Autodesk Inventor part; units mm, degrees
ref_plane "YZ Plane" through (0, 0, 0) normal (1, 0, 0) x (0, 1, 0)
ref_plane "XZ Plane" through (0, 0, 0) normal (0, 1, 0) x (-1, 0, 0)
ref_plane "XY Plane" through (0, 0, 0) normal (0, 0, 1) x (1, 0, 0)
sketch "Sketch1" plane through (0, 0, 0) normal (0, 0, 1) x (1, 0, 0)
  line L0 (1.5658, -2.5487) -> (1.5658, 2.559)
  arc A0 (1.5658, 2.559) -> (1.5824, -2.5487) centre (0, 0) ccw
  line L1 (1.5824, -2.5487) -> (1.5658, -2.5487)
  circle A1 centre (0, 0) radius 10
  circle A2 centre (0, 0) radius 3.1
  line L2 (1.7658, 2.5479) -> (1.7658, -2.5479)
  point P0 (0, 0)
  dimension "d0" = 20
  dimension "d1" = 6.2
  dimension "d2" = 0.2
extrude "Extrusion1" add sketch "Sketch1" against normal blind 10 contours A1 | A2 L2 picked at (2.2105, 0)
sketch "Sketch2" plane through (0, 0, 0) normal (0, 0, 1) x (1, 0, 0)
  circle A0 centre (0, 0) radius 3.1474
  circle A1 centre (0, 0) radius 10
extrude "Extrusion2" add sketch "Sketch2" along normal blind 15
sketch "Sketch3" plane through (0, 0, 15) normal (0, 0, 1) x (1, 0, 0)
  line L0 (7, 1.25) -> (-7, 1.25)
  line L1 (-7, 1.25) -> (-7, -1.25)
  line L2 (-7, -1.25) -> (7, -1.25)
  line L3 (7, -1.25) -> (7, 1.25)
  circle A0 centre (0, 0) radius 10
  dimension "d7" = 2.5
  dimension "d8" = 14
  dimension "d9" = 1.25
  dimension "d10" = 7
extrude "Extrusion3" add sketch "Sketch3" along normal blind 15
properties part number "RollerMotorCoupler"
Build history of the part. All positions in model axes, mm. A direction names the side the tool comes from. Round coordinates to 2 decimals unless told otherwise and drop trailing zeros. Write each loop counter-clockwise with the first axis right and the second up, starting at its lowest first coordinate (ties: lowest second). Pieces come first, ordered by that corner, then holes.
1) Band-saw the part on B-B, the plane x = 0. List the corners of the cut face in (y, z), and give its area (3 significant figures).
2) 3-axis set-ups, long thin cutter, end or side, ignore diameter. For faces 5 (the cylindrical face through (-3.144, -0.138, 7.395)), 6 (the flat face through (0, -1.25, 22)), 7 (the cylindrical face through (-3.1, 0.1, -4.9)): which of +Z, -Z, +X, -X, +Y, -Y reach the whole face in a straight line?
3) Band-saw the part on C-C, the plane z = 19. List the corners of the cut face in (x, y).
4) Band-saw the part on D-D, the plane x = -5. List the corners of the cut face in (y, z).
5) Pin check, flat tips, straight feed: pin 1 (12 mm diameter, centred on y = -5, z = 14.5, fed in from -X); pin 2 (1.2 mm diameter, centred on x = -4, y = 0.5, fed in from +Z); pin 3 (0.9 mm diameter, centred on x = 1, y = 2, fed in from -Z); pin 4 (6 mm diameter, centred on x = -6.5, z = 22.5, fed in from -Y). Stop position of each tip, or through.
6) Drill centre lines: probe 1 along Y at (x, z) = (0, 6.25); probe 2 along Z at (x, y) = (-6.75, -1); probe 3 along Y at (x, z) = (-2.25, 22.5). Where is each one in solid material? Low to high.
7) Mould opens along X. For faces 1 (the flat face through (2, 0, -10)), 2 (the cylindrical face through (-2.17, -9.76, 10.28)), 3 (the flat face through (-5, 0, 15)), 4 (the flat face through (5, 0, 15)) say: +X half, -X half, draft (parallel to the pull), parting line (faces both ways), or undercut.
8) Band-saw the part on A-A, the plane y = 0. List the corners of the cut face in (x, z).
Ans:
1. outline: (-10, -10) - (-3.1, -10) - (-3.1, 0) - (-3.15, 0) - (-3.15, 15) - (-1.25, 15) - (-1.25, 30) - (-10, 30) - close; (1.25, 15) - (3.15, 15) - (3.15, 0) - (3.1, 0) - (3.1, -10) - (10, -10) - (10, 30) - (1.25, 30) - close
1. area: 606 mm2
2. face 5: none
2. face 6: +Z
2. face 7: -Z
3. outline: circle Ø20 at (0, 0); hole (-7, -1.25) - (7, -1.25) - (7, 1.25) - (-7, 1.25) - close
4. outline: (-8.66, -10) - (8.66, -10) - (8.66, 30) - (1.25, 30) - (1.25, 15) - (-1.25, 15) - (-1.25, 30) - (-8.66, 30) - close
5. pin 1: stops at x = -10
5. pin 2: stops at z = 15
5. pin 3: stops at z = 15
5. pin 4: stops at y = -9.37
6. probe 1: y = -10 to -3.15, 3.15 to 10
6. probe 2: z = -10 to 15
6. probe 3: y = -9.74 to -1.25, 1.25 to 9.74
7. face 1: draft
7. face 2: parting line
7. face 3: undercut
7. face 4: undercut
8. outline: (-10, -10) - (-3.1, -10) - (-3.1, 0) - (-3.15, 0) - (-3.15, 15) - (-7, 15) - (-7, 30) - (-10, 30) - close; (1.77, -10) - (10, -10) - (10, 30) - (7, 30) - (7, 15) - (3.15, 15) - (3.15, 0) - (1.77, 0) - close
